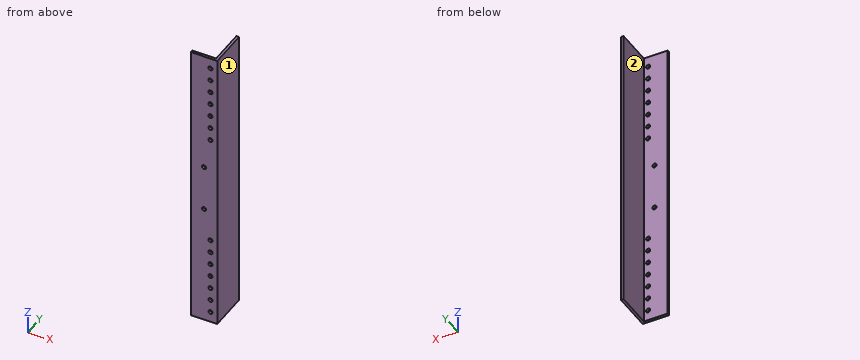
Autodesk Inventor part; units mm, degrees
ref_plane "YZ Plane" through (0, 0, 0) normal (1, 0, 0) x (0, 1, 0)
ref_plane "XZ Plane" through (0, 0, 0) normal (0, 1, 0) x (-1, 0, 0)
ref_plane "XY Plane" through (0, 0, 0) normal (0, 0, 1) x (1, 0, 0)
sketch "Szkic1" plane through (0, 0, 0) normal (0, 0, 1) x (1, 0, 0)
  line L0 (0, 0) -> (0, 30)
  line L1 (0, 30) -> (-2, 30)
  line L2 (-2, 30) -> (-2, 2)
  line L3 (-2, 2) -> (-20, 2)
  line L4 (-20, 2) -> (-20, 0)
  line L5 (-20, 0) -> (0, 0)
  dimension "d0" = 30
  dimension "d1" = 2
  dimension "d2" = 28
  dimension "d4" = 20
extrude "Wyciągnięcie proste1" add sketch "Szkic1" along normal mid plane 220
sketch "Szkic2" plane through (-20, 2, 110) normal (0, 1, 0) x (1, 0, 0)
  line L0 (18, 0) -> (0, 0)
  line L1 (20, 0) -> (20, 220)
  point P0 (20, 110)
  point P1 (14.8, 8.1)
  dimension "d7" = 8.1
  dimension "d8" = 5.2
hole "Otwór1" at (-5.2, 2, 101.9) direction (0, -1, 0) diameter 3.2 end through all
pattern_linear "Szyk prostokątny1" count 7 spacing 10 along (0, 0, -1) of "Otwór1"
mirror "Odbij1" about plane through (0, 0, 0) normal (0, 0, 1) of "Otwór1", "Szyk prostokątny1"
sketch "Szkic3" plane through (-20, 2, 110) normal (0, 1, 0) x (1, 0, 0)
  line L0 (24, 110) -> (-4, 110)
  line L1 (10, 127.5) -> (10, 92.5) construction
  line L2 (20, 220) -> (20, 0)
  point P0 (20, 110)
  point P1 (10, 110)
  dimension "d19" = 35
  dimension "d20" = 10
hole "Otwór2" at (-10, 2, -17.5) at (-10, 2, 17.5) direction (0, -1, 0) diameter 3.2 end through all
properties part number "bepf_podwozie_belka_glowna" material "Aluminium 6061"
Verification items for the finished model (mm, model axes). Face numbers are marked on the shaded views. A direction names the side the tool comes from. Coordinates: 2 decimals unless noted, no trailing zeros. Write each loop counter-clockwise with the first axis right and the second up, starting at its lowest first coordinate (ties: lowest second). Pieces come first, ordered by that corner, then holes. Notation, with made-up numbers: (78.25, 16) - (105.25, 16) arc R23 cw to (105.25, 46) - close; hole circle Ø3 at (33.25, -29.75). An arc over 180 degrees is marked (long way). Write item = value, one per line.
Q1. Material ranges on L1, parallel to X at y = 0.9, z = -81.9; L2, parallel to Z at x = -10, y = 1.2; L3, parallel to Z at x = -9.5, y = 1.5, recorded low to high. Write a range as from..to.
Answer:
L1 = -20..-6.8, -3.6..0
L2 = -110..-19.1, -15.9..15.9, 19.1..110
L3 = -110..-19.02, -15.98..15.98, 19.02..110
Q2. Cross-section at A-A (z = -6.5). Enter the section's corners in (x, y), plus the area to 3 significant figures.
Answer:
outline = (-20, 0) - (0, 0) - (0, 30) - (-2, 30) - (-2, 2) - (-20, 2) - close
area = 96.0 mm²
Q3. Cross-section at C-C (x = -16). Enter the section's corners in (y, z).
Answer:
outline = (0, -110) - (2, -110) - (2, 110) - (0, 110) - close
Q4. Cross-section at B-B (y = 18). Enter the section's corners in (x, z).
Answer:
outline = (-2, -110) - (0, -110) - (0, 110) - (-2, 110) - close
Q5. Access from +Z, -Z, +X, -X, +Y, -Y to the whole of each face (thin tool, end or side, straight path). Record for the marked faces 1 and 2.
Answer:
face_1 = +Z, -Z, +X, +Y, -Y
face_2 = +Z, -Z, -X, +Y
Q6. Go/stop test with flat-tipped pins: pin 1 Ø2.5 at (x, z) = (-10, 17.5) entering from -Y; pin 2 Ø3.5 at (x, z) = (-5.2, 91.9) entering from +Y; pin 3 Ø5 at (y, z) = (21.5, 41.5) entering from -X. Record where each tip stops, or that it passes through.
Answer:
pin_1 = through
pin_2 = 2
pin_3 = -2
